The listing builds one solid part. Answer for the finished solid, in the listing's coordinates (mm). A direction names the side the tool comes from. Give positions to 0.01 mm unless a question says otherwise; leave off trailing zeros. Loops run counter-clockwise (first coordinate to the right, second up) from the corner with the lowest first, then second, coordinate; pieces in that order, holes last. Notation, with made-up numbers: M 21,67.5 L 39,67.5 A14 cw 39,92.5 Z; hole C 87.5,-23.5 d10. An arc over 180 degrees is marked long. Use one line per item in the form item = value. Start each with the question number.
1. The mould has two halves that part along X. Classify faces 5 (the face through (8.44, 9.33, 4.96)), 6 (the face through (5.111, -4.094, 3.944)), 7 (the face through (-1, 35, 1)): released by +X, released by -X, zero draft, split by the parting line, or undercut.
2. Each of these flat-tipped pins is pushed along its axis until it touches: pin 1 Ø2 at (x, z) = (1.5, 9.5) entering from -Y; pin 2 Ø3 at (x, y) = (5.27, -5.33) entering from +Z; pin 3 Ø2 at (x, y) = (5.33, 5.27) entering from +Z; pin 4 Ø2 at (y, z) = (14.5, 6) entering from -X. Where does it stop, or does it pass through?
3. The part is cut by section D-D (z = 4.5). Write down the section's boundary in (x, y).
4. Straight lines are drawn through the part: line 1 (Y direction, x = 0, z = 6.4); line 2 (Y direction, x = 0.75, z = 5.75); line 3 (Y direction, x = 5.25, z = 7). For each, find the intervals that lie inside material, in ascending order. Write a range as from..to.
5. The part is cut by section B-B (x = 0). Give the number of separate pieces and of enclosed holes in the cut face, and give its area (3 significant figures).
6. The part is cut by section A-A (z = 9.25). Write down the section's boundary in (x, y), and give its area (3 significant figures).
7. For faces 1 (the face through (7.43, 22.88, 5.94)), 2 (the face through (3, 3, 3)), 3 (the face through (7.448, 8.871, 1.014)), 4 (the face through (3, -3, 5)), determine the directions among +Z, -Z, +X, -X, +Y, -Y from which every point of the face is accessible in a straight line to the end or side of a thin tool.
8. The part is cut by section C-C (y = 0). Write down the section's boundary in (x, z).
from build123d import *
from OCP.BRepFilletAPI import BRepFilletAPI_MakeChamfer

# Parameters (mm, degrees)
SKETCH_1_R          = 1.25
SKETCH_1_R_2        = 4
SKETCH_1_R_3        = 2.3
EXTRUDE_2_DEPTH     = 8
CHAMFER_1_SIZE      = 5
EXTRUDE_3_DEPTH     = 2
SKETCH_3_R          = 2.3
CUT_EXTRUDE_1_DEPTH = 7
CUT_EXTRUDE_2_DEPTH = 10
CHAMFER_2_SIZE      = 5
CHAMFER_2_SIZE2     = 6.028089953
CHAMFER_2_SIZE2_2   = 6.039479554
CHAMFER_3_SIZE      = 2
SKETCH_5_R          = 5.05
CUT_EXTRUDE_3_DEPTH = 3
CUT_EXTRUDE_START   = -3
SKETCH_6_R          = 5.05
CUT_EXTRUDE_4_DEPTH = 3
FILLET_1_R          = 0.5
SKETCH_7_R          = 4.05
CUT_EXTRUDE_5_DEPTH = 3
FILLET_2_R          = 0.5


with BuildPart() as part:
    # 草图1 → 凸台-拉伸2 (new body)
    with BuildSketch(Plane.XY):
        Polygon((8.5, 36), (12.5, 11.216882722), (12.5, -12), (-12.5, -12), (-12.5, 11), (-8.5, 36), align=None)
        with Locations((-5.273420283, 5.333014019)):
            Circle(SKETCH_1_R, mode=Mode.SUBTRACT)
        with Locations((5.333014019, 5.273420283)):
            Circle(SKETCH_1_R, mode=Mode.SUBTRACT)
        with Locations((5.273420283, -5.333014019)):
            Circle(SKETCH_1_R, mode=Mode.SUBTRACT)
        with Locations((-5.333014019, -5.273420283)):
            Circle(SKETCH_1_R, mode=Mode.SUBTRACT)
        Circle(SKETCH_1_R_2, mode=Mode.SUBTRACT)
        with Locations((0, 29)):
            Circle(SKETCH_1_R_3, mode=Mode.SUBTRACT)
    extrude(amount=EXTRUDE_2_DEPTH)

    # 倒角1
    chamfer_1_edges = [part.edges().sort_by_distance(p)[0] for p in [
        (12.5, -12, 4),
        (-12.5, -12, 4),
    ]]
    chamfer(chamfer_1_edges, length=CHAMFER_1_SIZE)

    # 草图2 → 凸台-拉伸3 (add)
    with BuildSketch(Plane.XY.offset(8)):
        Polygon((-10.577137485, 23.017890722), (-5.61376382, 21), (5.631941325, 21), (10.595314989, 23.017890722), (8.5, 36), (-8.5, 36), align=None)
    extrude(amount=EXTRUDE_3_DEPTH)

    # 草图3 → 切除-拉伸1 (cut)
    with BuildSketch(Plane(origin=(0, 0, 8), x_dir=(-1, 0, 0), z_dir=(0, 0, -1))):
        with Locations(Location((0, 29, 0), (0, 0, 180))):
            Circle(SKETCH_3_R)
    extrude(amount=-CUT_EXTRUDE_1_DEPTH, mode=Mode.SUBTRACT)

    # 草图4 → 切除-拉伸2 (cut)
    with BuildSketch(Plane(origin=(0, 0, 0), x_dir=(-1, 0, 0), z_dir=(0, 0, -1))):
        Polygon((-10.275402162, 25), (-4.5, 20.700412405), (-4.5, 12.565758544), (-12.5, 6), (-12.5, 11.216882722), align=None)
    extrude(amount=-CUT_EXTRUDE_2_DEPTH, mode=Mode.SUBTRACT)

    # 倒角2: one chamfer whose edges measure the first distance from different faces: ONE call of the kernel's chamfer builder (chamfer() names one face for all edges)
    chamfer_2_edges_1 = [part.edges().sort_by_distance(p)[0] for p in [
        (-8.5, 36, 5),
    ]]
    chamfer_2_side_1 = [part.faces().sort_by_distance(p)[0] for p in [
        (0, 36, 5),
    ]]
    chamfer_2_edges_2 = [part.edges().sort_by_distance(p)[0] for p in [
        (8.5, 36, 5),
    ]]
    chamfer_2_side_2 = [part.faces().sort_by_distance(p)[0] for p in [
        (9.387701081, 30.5, 5),
    ]]
    chamfer_2 = BRepFilletAPI_MakeChamfer(part.part.solid().wrapped)
    for e in chamfer_2_edges_1:
        chamfer_2.Add(CHAMFER_2_SIZE, CHAMFER_2_SIZE2, e.wrapped, chamfer_2_side_1[0].wrapped)  # the first distance lies on this face
    for e in chamfer_2_edges_2:
        chamfer_2.Add(CHAMFER_2_SIZE, CHAMFER_2_SIZE2_2, e.wrapped, chamfer_2_side_2[0].wrapped)  # the first distance lies on this face
    add(Compound.cast(chamfer_2.Shape()), mode=Mode.REPLACE)

    # 倒角3
    chamfer_3_edges = [part.edges().sort_by_distance(p)[0] for p in [
        (-0.519739777, 36, 0),
        (-10.976190476, 20.523809524, 0),
        (-6.476190476, 33.023809524, 0),
        (5.878605618, 33.531939841, 0),
        (0, -12, 0),
        (12.5, -0.5, 0),
        (10, -9.5, 0),
        (-10, -9.5, 0),
        (9.786046476, 28.031939841, 0),
        (-12.5, 2, 0),
        (8.5, 9.282879272, 0),
        (4.5, 16.633085475, 0),
        (7.387701081, 22.850206203, 0),
    ]]
    chamfer(chamfer_3_edges, length=CHAMFER_3_SIZE)

    # 草图5 → 切除-拉伸3 (cut)
    with BuildSketch(Plane(origin=(0, 0, 0), x_dir=(-1, 0, 0), z_dir=(0, 0, -1))):
        Circle(SKETCH_5_R)
    extrude(amount=-CUT_EXTRUDE_3_DEPTH, mode=Mode.SUBTRACT)

    # 草图6 → 切除-拉伸4 (cut)
    with BuildSketch(Plane.XY.offset(8).offset(CUT_EXTRUDE_START)):
        with Locations(Location((0, 0, 0), (0, 0, 180))):
            Circle(SKETCH_6_R)
    extrude(amount=CUT_EXTRUDE_4_DEPTH, mode=Mode.SUBTRACT)

    # 圆角1
    fillet_1_edges = [part.edges().sort_by_distance(p)[0] for p in [
        (5.05, 0, 0),
        (5.05, 0, 8),
    ]]
    fillet(fillet_1_edges, radius=FILLET_1_R)

    # 草图7 → 切除-拉伸5 (cut)
    with BuildSketch(Plane(origin=(0, 0, 0), x_dir=(-1, 0, 0), z_dir=(0, 0, -1))):
        with Locations((0, 29)):
            Circle(SKETCH_7_R)
    extrude(amount=-CUT_EXTRUDE_5_DEPTH, mode=Mode.SUBTRACT)

    # 圆角2
    fillet_2_edges = [part.edges().sort_by_distance(p)[0] for p in [
        (4.05, 29, 0),
    ]]
    fillet(fillet_2_edges, radius=FILLET_2_R)


solid = part.part
Derived:
q1.face_5 = released by +X
q1.face_6 = undercut
q1.face_7 = zero draft
q2.pin_1 = 21
q2.pin_2 = 8
q2.pin_3 = through
q2.pin_4 = -12.1
q3.outline = M -12.5,-7 L -7.5,-12 L 7.5,-12 L 12.5,-7 L 12.5,6 L 4.5,12.57 L 4.5,20.7 L 10.28,25 L 9.3,31.06 L 2.46,36 L -3.5,36 L -9.45,30.05 L -12.5,11 Z; hole C -5.33,-5.27 d2.5; hole C -5.27,5.33 d2.5; hole C 0,0 d8; hole C 0,29 d4.6; hole C 5.27,-5.33 d2.5; hole C 5.33,5.27 d2.5
q4.line_1 = -12..-5.05, 5.05..26.7, 31.3..36
q4.line_2 = -12..-4.99, 4.99..26.83, 31.17..36
q4.line_3 = -12..-6.58, -4.08..4.03, 6.52..11.95, 21.26..33.99
q5.separate_pieces = 3
q5.enclosed_holes = 0
q5.area = 277 mm2
q6.outline = M -10.58,23.02 L -5.61,21 L 4.9,21 L 10.28,25 L 9.3,31.06 L 2.46,36 L -3.5,36 L -9.45,30.05 Z; hole C 0,29 d4.6
q6.area = 227 mm2
q7.face_1 = +Z, -Z, +X
q7.face_2 = -Z
q7.face_3 = -Z, +X
q7.face_4 = +Z
q8.outline = M -12.5,2 L -10.5,0 L -5.55,0 A0.5 ccw -5.05,0.5 L -5.05,3 L -4,3 L -4,5 L -5.05,5 L -5.05,7.5 A0.5 ccw -5.55,8 L -12.5,8 Z; M 4,3 L 5.05,3 L 5.05,0.5 A0.5 ccw 5.55,0 L 10.5,0 L 12.5,2 L 12.5,8 L 5.55,8 A0.5 ccw 5.05,7.5 L 5.05,5 L 4,5 Z
